The model under review builds one solid part; all positions refer to its coordinate system, in mm. A direction names the side the tool comes from. Give positions to 0.01 mm unless a question says otherwise; leave off trailing zeros. Order: outer loops, then holes, each group sorted by start corner. A loop starts at its lowest first (then second) coordinate and runs counter-clockwise, first axis right, second up. Notation, with made-up numbers: (65, 8) -> (70, 8) arc R24 ccw to (70, 38) -> close; hole circle Ø9 at (16.5, -30). An arc over 180 degrees is marked (long way). Answer as a JSON object with one key per item and string values. Group by question number.
from build123d import *

# Parameters (mm, degrees)
F1_W     = 154.501944
F1_H     = 150.962084
F2_DEPTH = 77.229418
F3_T     = -2.54
F4_W     = 149.421944
F4_H     = 3.407732
F5_DEPTH = 59.480889


with BuildPart() as f2:
    # F1 (on face) → F2 (new body)
    with BuildSketch(Plane.XZ):
        Rectangle(F1_W, F1_H)
    extrude(amount=F2_DEPTH)

    # F3
    f3_openings = [f2.faces().sort_by_distance(p)[0] for p in [
        (0, -77.229418, 0),
    ]]
    offset(amount=F3_T, openings=f3_openings)

    # F4 (on face) → F5 (join)
    with BuildSketch(Plane.XZ.offset(2.54)):
        with Locations((0, -19.762568)):
            Rectangle(F4_W, F4_H)
    extrude(amount=F5_DEPTH)


solid = f2.part
1. Draft analysis for pull direction Z (two halves, no side actions). For faces 1 (the flat face through (-1, -38, 75.481)), 2 (the flat face through (-75, -77.229, 34)), 3 (the flat face through (-1, -38, -75.481)), 4 (the flat face through (-1, -32, -18.059)), state which applies: pulls with the +Z half, pulls with the -Z half, needs draft (parallel to the pull), parting line crosses it, or undercut.
2. Take a section at D-D on z = 53. Give the boundary of the cut face in (x, y).
3. Take a section at A-A on y = -36. Give the boundary of the cut face in (x, z).
4. Machinability: for faces 5 (the flat face through (-1, -32, -21.466)), 6 (the flat face through (-77.251, -38, -1)), which of the approach directions +Z, -Z, +X, -X, +Y, -Y give a long, thin tool a straight path to every point of the face, cutting with its end or side? Answer none if there is none.
5. For probe 1 along Z at (x, y) = (-32, -50); probe 2 along X at (y, z) = (-74, 57); probe 3 along Y at (x, z) = (32, 55), list the stretches that pass through material, from the lowest coordinate up. Write a range as [from, to].
6. Take a section at B-B on x = 30. Give the boundary of the cut face in (y, z).
7. Take a section at C-C on y = -64.5. Give the boundary of the cut face in (x, z).
8. For pin 1 (1.5 mm diameter, centred on x = -49.5, z = -52, fed in from -Y); pin 2 (2.5 mm diameter, centred on x = 34, z = -19, fed in from -Y), all flat-tipped, find the tip position at first contact; note any pin that passes through.
Checks:
{
 "1": {"face 1": "pulls with the +Z half", "face 2": "needs draft", "face 3": "pulls with the -Z half", "face 4": "undercut"},
 "2": {"outline": "(-77.25, -77.23) -> (-74.71, -77.23) -> (-74.71, -2.54) -> (74.71, -2.54) -> (74.71, -77.23) -> (77.25, -77.23) -> (77.25, 0) -> (-77.25, 0) -> close"},
 "3": {"outline": "(-77.25, -75.48) -> (77.25, -75.48) -> (77.25, 75.48) -> (-77.25, 75.48) -> close; hole (-74.71, -72.94) -> (74.71, -72.94) -> (74.71, -21.47) -> (-74.71, -21.47) -> close; hole (-74.71, -18.06) -> (74.71, -18.06) -> (74.71, 72.94) -> (-74.71, 72.94) -> close"},
 "4": {"face 5": "-Y", "face 6": "+Z, -Z, -X, +Y, -Y"},
 "5": {"probe 1": "z = [-75.48, -72.94], [-21.47, -18.06], [72.94, 75.48]", "probe 2": "x = [-77.25, -74.71], [74.71, 77.25]", "probe 3": "y = [-2.54, 0]"},
 "6": {"outline": "(-77.23, -75.48) -> (0, -75.48) -> (0, 75.48) -> (-77.23, 75.48) -> (-77.23, 72.94) -> (-2.54, 72.94) -> (-2.54, -18.06) -> (-62.02, -18.06) -> (-62.02, -21.47) -> (-2.54, -21.47) -> (-2.54, -72.94) -> (-77.23, -72.94) -> close"},
 "7": {"outline": "(-77.25, -75.48) -> (77.25, -75.48) -> (77.25, 75.48) -> (-77.25, 75.48) -> close; hole (-74.71, -72.94) -> (74.71, -72.94) -> (74.71, 72.94) -> (-74.71, 72.94) -> close"},
 "8": {"pin 1": "stops at y = -2.54", "pin 2": "stops at y = -62.02"}
}
